Could you check a few things on this drawing? It's one solid part, dimensions in mm from its lowest x, y, z. Round coordinates to 2 decimals unless told otherwise and drop trailing zeros. Write each loop counter-clockwise with the first axis right and the second up, starting at its lowest first coordinate (ties: lowest second). Pieces come first, ordered by that corner, then holes. Notation, with made-up numbers: (37, -28.5) -> (70, -28.5) arc R23 cw to (70, -0.5) -> close; hole circle Ø9 at (86.25, 64). An arc over 180 degrees is marked (long way). Return JSON: item names as keys, results as strings.
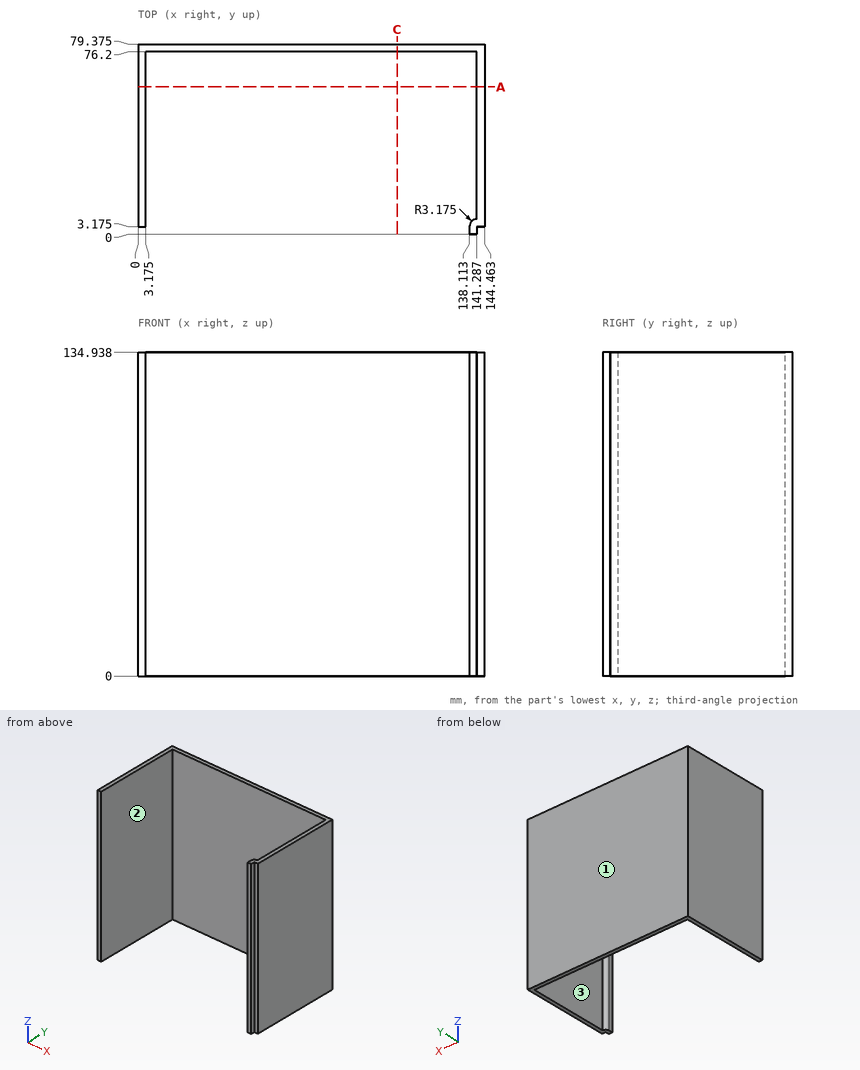
1) Thinking about a two-plate mould opening in Y: for the marked faces 1, 2 and 3, which applies, pulls with the +Y half, pulls with the -Y half, needs draft (parallel to the pull), parting line crosses it, or undercut?
Return value:
{"face 1": "pulls with the +Y half", "face 2": "needs draft", "face 3": "undercut"}
2) I want a section at A-A, the plane y = 61.5. Please give me the cut outline in (x, z) (1 decimal).
Return value:
{"outline": "(0, 0) -> (3.2, 0) -> (3.2, 134.9) -> (0, 134.9) -> close; (141.3, 0) -> (144.5, 0) -> (144.5, 134.9) -> (141.3, 134.9) -> close"}
3) If I drill on probe 1 along X at (y, z) = (10, 70) (1 decimal); probe 2 along Y at (x, z) = (122, 77) (1 decimal), over which ranges is the centre line in solid material (lowest first)? Write a range as [from, to].
Return value:
{"probe 1": "[0, 3.2], [141.3, 144.5]", "probe 2": "[76.2, 79.4]"}
4) I want a section at C-C, the plane x = 108. Please give me the cut outline in (y, z) (1 decimal).
Return value:
{"outline": "(76.2, 0) -> (79.4, 0) -> (79.4, 134.9) -> (76.2, 134.9) -> close"}
5) Will these pins go through, and if not, where does the flat tip stop? pin 1 Ø1.6 at (y, z) = (2, 90) entering from +X; pin 2 Ø3.5 at (x, z) = (1, 79) entering from -Y (1 decimal); pin 3 Ø10 at (x, z) = (52, 36.5) entering from -Y.
Return value:
{"pin 1": "x = 141.29", "pin 2": "y = 3.2", "pin 3": "y = 76.2"}
